Source: CAD feature listing. Evaluate the final solid. Frame: model axes, mm. Face numbers are marked on the shaded views. A direction names the side the tool comes from. Round coordinates to 2 decimals unless told otherwise and drop trailing zeros. Order: outer loops, then holes, each group sorted by start corner. A loop starts at its lowest first (then second) coordinate and runs counter-clockwise, first axis right, second up. Notation, with made-up numbers: (57, 6) - (71, 6) arc R9 cw to (71, 20) - close; hole circle Ø2 at (-1.75, 22.5). An arc over 180 degrees is marked (long way). Use one line per item in the form item = value. Start each with the question number.
Q1. Pin query (flat end, axial travel): pin 1 Ø10 at (x, y) = (-197, 1.5) entering from +Z; pin 2 Ø1 at (y, z) = (-18.5, 8.5) entering from -X; pin 3 Ø6 at (x, y) = (-173.5, -24) entering from -Z. Return the tip coordinate at first contact, or that it passes through.
Q2. Ray query, line 1 (Z direction, x = -239, y = 0); line 2 (X direction, y = -14, z = 13.5); line 3 (Z direction, x = -176, y = 10). Return the intervals inside material, ascending. Write a range as [from, to].
Q3. Set-up query: the marked faces 1 and 2. Return all of +Z, -Z, +X, -X, +Y, -Y with unobstructed straight access to the full face (end or side cutting, diameter ignored); none if empty.
Q4. Cut plane A-A, the plane x = -265. Return the cut outline in (y, z).
Q5. Cut plane B-B, the plane x = -49. Return the cut outline in (y, z).
from build123d import *


# Not quite as in the source:
# - ends of sketch curves that miss each other by under 0.0002 mm in the source are joined
# - the dataset's text gives a spline's control points without its knots; the knots are read off the source's solid


with BuildPart() as f1:
    # F0 (on Top) → F1 (revolve)
    with BuildSketch(Plane.XY):
        with BuildLine():
            ThreePointArc((-285.75, -11.43), (-285.5490287786, -12.167016937), (-285.0017514707, -12.7))
            Line((-285.0017514707, -12.7), (-216.5853927097, -12.7))
            ThreePointArc((-216.5853927097, -12.7), (-209.8052797295, -13.6216408234), (-203.5172005218, -16.3196796869))
            Line((-203.5172005218, -16.3196796869), (-171.3760702521, -35.6043578488))
            ThreePointArc((-171.3760702521, -35.6043578488), (-164.8344445945, -38.3712151601), (-157.7824732637, -39.2186028951))
            Line((-157.7824732637, -39.2186028951), (19.05, -35.56))
            add(Edge.make_bspline(
                [(19.05, -35.56), (18.8199370568, -30.7601188197), (-1.2317807445, -20.8787296757), (0.1635549587, -4.0029242831), (-5.1918e-06, -1.9625883677), (0, 0)],
                knots=[0, 0, 0, 0, 0.4507733435, 0.8068049822, 1, 1, 1, 1], degree=3))
            Line((0, 0), (-2.54, 0))
            add(Edge.make_bspline(
                [(14.8285794135, -33.1067947702), (14.5353050036, -32.7990607261), (13.8691865137, -32.1447406693), (12.2944674544, -30.73758966), (9.9695334737, -28.8275639769), (7.4490348824, -26.7626250066), (5.4570185152, -25.0088190546), (4.0093053584, -23.6366363216), (2.641510283, -22.1980089148), (1.5988268496, -20.9351240128), (0.8394327936, -19.8719511734), (0.1492382006, -18.7893744625), (-0.5810765462, -17.4218736538), (-1.2672380096, -15.7774032099), (-1.9564088602, -13.6109085126), (-2.4520800573, -11.0014246266), (-2.6128292518, -8.638851289), (-2.627993734, -6.9624293235), (-2.6035900901, -5.8300997647), (-2.5708007223, -5.0090073669), (-2.547044183, -4.4386671163), (-2.5331221367, -4.0633936667), (-2.5236240841, -3.723792553), (-2.5156422476, -3.3057754423), (-2.5131648633, -2.8291110855), (-2.5181696061, -2.2621652533), (-2.530667923, -1.4312861782), (-2.5400016792, -0.6509680927), (-2.54, 0)],
                knots=[0.1260546343, 0.1260546343, 0.1260546343, 0.1260546343, 0.15625, 0.1875, 0.25, 0.3125, 0.34375, 0.375, 0.40625, 0.4375, 0.453125, 0.46875, 0.5, 0.53125, 0.5625, 0.625, 0.6875, 0.71875, 0.75, 0.78125, 0.796875, 0.8125, 0.828125, 0.84375, 0.875, 0.90625, 0.9375, 0.999999785, 0.999999785, 0.999999785, 0.999999785], degree=3))
            Line((14.8285794135, -33.1067947702), (-157.8350137437, -36.6791463592))
            ThreePointArc((-157.8350137437, -36.6791463592), (-164.1817879415, -35.9164973976), (-170.0692510333, -33.4263258174))
            Line((-170.0692510333, -33.4263258174), (-202.210381303, -14.1416476556))
            ThreePointArc((-202.210381303, -14.1416476556), (-209.1272684315, -11.1738049058), (-216.5853927097, -10.16))
            Line((-216.5853927097, -10.16), (-285.0017514707, -10.16))
            ThreePointArc((-285.0017514707, -10.16), (-285.5490287786, -10.692983063), (-285.75, -11.43))
        make_face()
    revolve(axis=Axis((-142.875, 0, 0), (-1, 0, 0)))


solid = f1.part
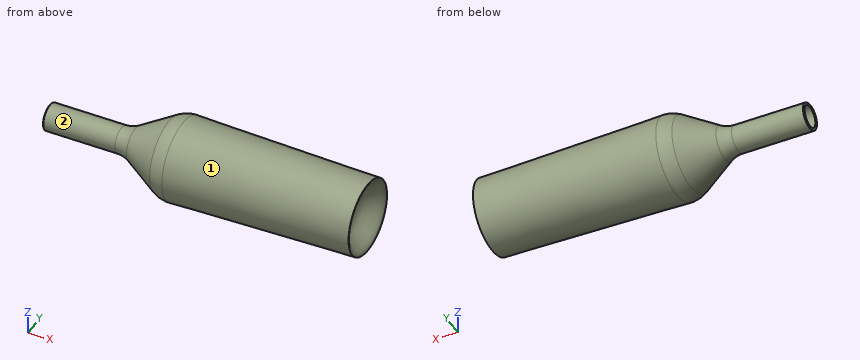
Completed:
q1.pin_1 = 23.19
q1.pin_2 = -197.62
q1.pin_3 = -28.09
q2.line_1 = [-12.7, -10.16], [10.16, 12.7]
q2.line_2 = [-198.3, -193.37], [0.57, 3.68]
q2.line_3 = [-31.27, -28.14], [28.14, 31.27]
q3.face_1 = +X
q3.face_2 = -X
q4.outline = circle Ø25.4 at (0, 0); hole circle Ø20.32 at (0, 0)
q5.outline = circle Ø73.94 at (0, 0); hole circle Ø68.85 at (0, 0)
